from build123d import *

# Parameters (mm, degrees)
BOSS_EXTRUDE1_DEPTH                          = 55
CSK_FOR_M3_HEX_SOCKET_COUNTERSUNK_CA_2_COUNT = 2
CSK_FOR_M3_HEX_SOCKET_COUNTERSUNK_CA_2_PITCH = 32


with BuildPart() as part:
    # Sketch2 → Boss-Extrude1 (new body)
    with BuildSketch(Plane.XY):
        Polygon((-11, 0), (11, 0), (11, 4.5), (9.5, 6), (5.15, 6), (8.15, 3), (-8.15, 3), (-5.15, 6), (-9.5, 6), (-11, 4.5), align=None)
    extrude(amount=BOSS_EXTRUDE1_DEPTH)

    # Sketch4 → CSK for M3 Hex Socket Countersunk Cap Screw1 (revolve, cut)
    with BuildSketch(Plane(origin=(0, 3, 11.5), x_dir=(0, 0, 1), z_dir=(1, 0, 0))):
        Polygon((0, 0), (0, 3), (1.8, 3), (1.8, 1.56), (3.36, 0), align=None)
    csk_for_m3_hex_socket_countersunk_cap_sc = revolve(axis=Axis((0, 9.35, 11.5), (0, -1, 0)), mode=Mode.SUBTRACT)

    # CSK for M3 Hex Socket Countersunk Ca 2: CSK for M3 Hex Socket Countersunk Cap Screw1 ×2
    with Locations(*[(0, 0, i * CSK_FOR_M3_HEX_SOCKET_COUNTERSUNK_CA_2_PITCH) for i in range(1, CSK_FOR_M3_HEX_SOCKET_COUNTERSUNK_CA_2_COUNT)]):
        add(csk_for_m3_hex_socket_countersunk_cap_sc, mode=Mode.SUBTRACT)


solid = part.part
CAD build for the part. Positions are in the model's coordinates, mm. A direction names the side the tool comes from. Coordinates: 2 decimals unless noted, no trailing zeros. Order: outer loops, then holes, each group sorted by start corner. A loop starts at its lowest first (then second) coordinate and runs counter-clockwise, first axis right, second up.
Item 1: Band-saw the part on D-D on z = 4. List the corners of the cut face in (x, y), plus the area to 4 significant figures.
Check sheet entries:
outline: (-11, 0) - (11, 0) - (11, 4.5) - (9.5, 6) - (5.15, 6) - (8.15, 3) - (-8.15, 3) - (-5.15, 6) - (-9.5, 6) - (-11, 4.5) - close
area: 89.85 mm2
Item 2: Two-plate mould, pull along Y, no slides. Class faces 1 (the face through (7, 6, 27)), 2 (the face through (-0.541, 0.73, 45.217)), 3 (the face through (-6.67, 4.48, 27.12)): +Y half, -Y half, draft (parallel to the pull), parting line (faces both ways), or undercut.
Check sheet entries:
face 1: +Y half
face 2: draft
face 3: undercut
Item 3: Band-saw the part on A-A on x = 0. List the corners of the cut face in (y, z), plus the area to 3 significant figures.
Check sheet entries:
outline: (0, 0) - (3, 0) - (3, 8.14) - (1.44, 9.7) - (0, 9.7) - close; (0, 13.3) - (1.44, 13.3) - (3, 14.86) - (3, 40.14) - (1.44, 41.7) - (0, 41.7) - close; (0, 45.3) - (1.44, 45.3) - (3, 46.86) - (3, 55) - (0, 55) - close
area: 139 mm2
Item 4: Band-saw the part on C-C on y = 2. List the corners of the cut face in (x, z).
Check sheet entries:
outline: (-11, 0) - (11, 0) - (11, 55) - (-11, 55) - close; hole circle Ø4.72 at (0, 11.5); hole circle Ø4.72 at (0, 43.5)
Item 5: Drill centre lines: L1, parallel to Z at x = 0, y = 0.9; L2, parallel to X at y = 0.45, z = 11.5; L3, parallel to Y at x = 0.25, z = 22.5. Where is each one in solid material? Low to high.
Check sheet entries:
L1: z = 0 to 9.7, 13.3 to 41.7, 45.3 to 55
L2: x = -11 to -1.8, 1.8 to 11
L3: y = 0 to 3
Item 6: 3-axis set-ups, long thin cutter, end or side, ignore diameter. For faces 4 (the face through (-10.2, 5.3, 27.1)), 5 (the face through (0, 3, 27)): which of +Z, -Z, +X, -X, +Y, -Y reach the whole face in a straight line?
Check sheet entries:
face 4: +Z, -Z, -X, +Y
face 5: +Z, -Z
Item 7: Pin check, flat tip, straight feed: pin 1 Ø5 at (x, z) = (-2.5, 37) entering from +Y. Stop position of the tip, or through.
Check sheet entries:
pin 1: stops at y = 3
Item 8: Band-saw the part on B-B on z = 11.5. List the corners of the cut face in (x, y).
Check sheet entries:
outline: (-11, 0) - (-1.8, 0) - (-1.8, 1.44) - (-3.36, 3) - (-8.15, 3) - (-5.15, 6) - (-9.5, 6) - (-11, 4.5) - close; (1.8, 0) - (11, 0) - (11, 4.5) - (9.5, 6) - (5.15, 6) - (8.15, 3) - (3.36, 3) - (1.8, 1.44) - close
